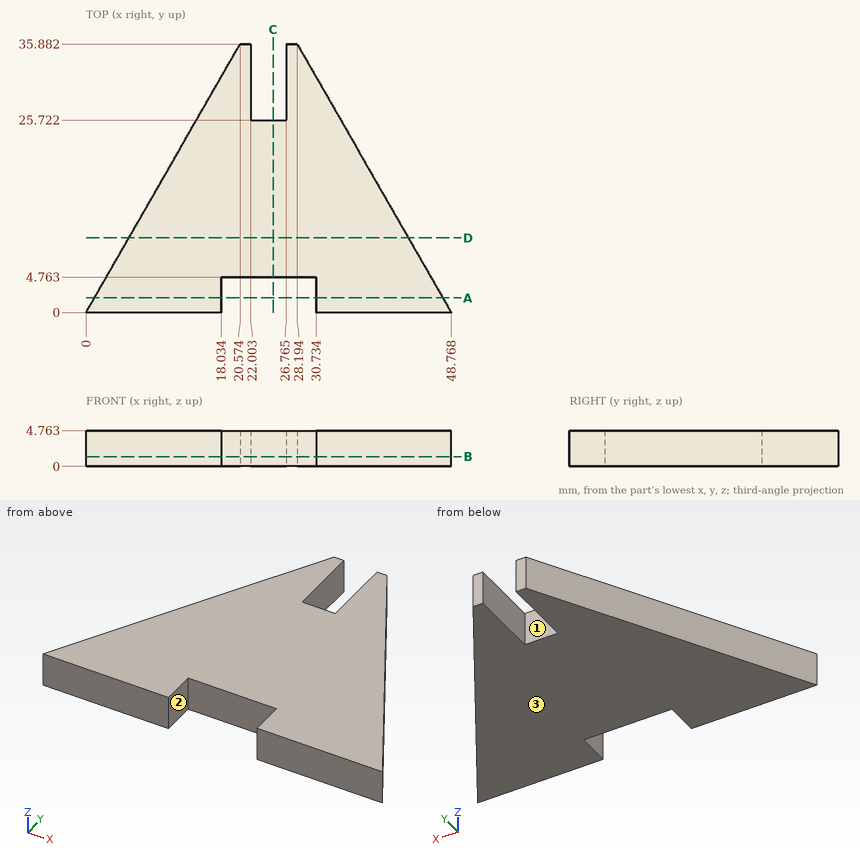
Can you work these out from the drawing? Everything is in mm from the part's minimum corner. A direction names the side the tool comes from. Give positions to 0.01 mm unless a question says otherwise; leave off trailing zeros. Order: outer loops, then holes, each group sorted by start corner. A loop starts at its lowest first (then second) coordinate and runs counter-clockwise, first axis right, second up.
Item 1: I'm going to push flat-ended pins straight in: pin 1 (2.5 mm diameter, centred on x = 23.5, z = 1.5, fed in from +Y); pin 2 (2 mm diameter, centred on x = 18.5, z = 4, fed in from +Y); pin 3 (1.5 mm diameter, centred on y = 17.5, z = 3.5, fed in from +X) (1 decimal). Where does each tip first touch, or does it pass through?
Item 2: If we section it at B-B, the plane z = 1.3: Write out the boundary of the cut face in (x, y) (1 decimal), plus the area to 3 significant figures.
Item 3: For the marked faces 1, 2 and 3, which set-ups out of +Z, -Z, +X, -X, +Y, -Y let a thin tool reach every point of the face, with its end or its side?
Item 4: If we section it at A-A, the plane y = 2: Write out the boundary of the cut face in (x, z) (1 decimal), plus the area to 3 significant figures.
Item 5: I need wall thicknesses on line 1 (X direction, y = 29, z = 1.85) (1 decimal); line 2 (X direction, y = 29.5, z = 3.65) (1 decimal); line 3 (Y direction, x = 25, z = 2.3). Which ranges of each line are inside material? Lowest first, please.
Item 6: If we section it at D-D, the plane y = 10: Write out the boundary of the cut face in (x, z) (1 decimal).
Item 7: If we section it at C-C, the plane x = 25: Write out the boundary of the cut face in (y, z).
Values:
1. pin 1: stops at y = 25.72
1. pin 2: stops at y = 34.01
1. pin 3: stops at x = 39.2
2. outline: (0, 0) - (18, 0) - (18, 4.8) - (30.7, 4.8) - (30.7, 0) - (48.8, 0) - (28.2, 35.9) - (26.8, 35.9) - (26.8, 25.7) - (22, 25.7) - (22, 35.9) - (20.6, 35.9) - close
2. area: 903 mm2
3. face 1: +Z, -Z, +Y
3. face 2: +Z, -Z, -Y
3. face 3: -Z, +X, -X, +Y, -Y
4. outline: (1.1, 0) - (18, 0) - (18, 4.8) - (1.1, 4.8) - close; (30.7, 0) - (47.6, 0) - (47.6, 4.8) - (30.7, 4.8) - close
4. area: 161 mm2
5. line 1: x = 16.6 to 22, 26.8 to 32.1
5. line 2: x = 16.9 to 22, 26.8 to 31.9
5. line 3: y = 4.76 to 25.72
6. outline: (5.7, 0) - (43, 0) - (43, 4.8) - (5.7, 4.8) - close
7. outline: (4.76, 0) - (25.72, 0) - (25.72, 4.76) - (4.76, 4.76) - close
